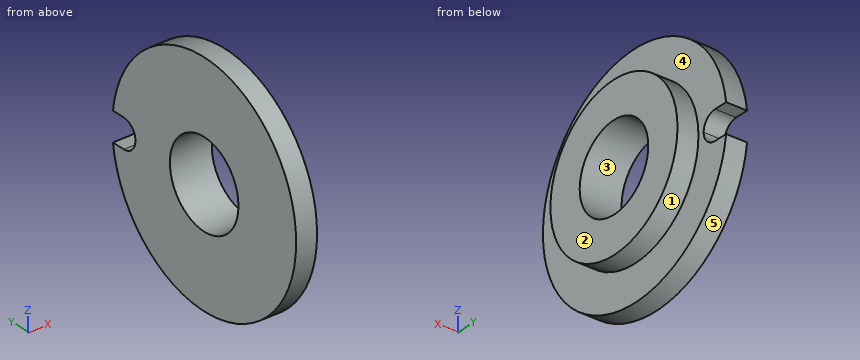
```python
from build123d import *

# Parameters (mm, degrees)
F0_R     = 11
F0_R_2   = 7.6
F1_DEPTH = 2
F2_DEPTH = 2
F3_R     = 4.1
F4_DEPTH = 25
F6_DEPTH = 5


# Not quite as in the source:
# - a feature names something its author has since deleted; it is built from what else it names


with BuildPart() as f1:
    # F0 (on Right) → F1 (new body)
    with BuildSketch(Plane.YZ):
        Circle(F0_R)
        Circle(F0_R_2, mode=Mode.SUBTRACT)
        Circle(F0_R_2)
    extrude(amount=-F1_DEPTH)

    # F0 (on Right) → F2 (join)
    with BuildSketch(Plane.YZ):
        Circle(F0_R_2)
    extrude(amount=F2_DEPTH)

    # F3 (on face) → F4 (cut)
    with BuildSketch(Plane(origin=(-2, 0, 0), x_dir=(0, -1, 0), z_dir=(-1, 0, 0))):
        Circle(F3_R)
    extrude(amount=-F4_DEPTH, mode=Mode.SUBTRACT)

    # F5 (on face) → F6 (cut)
    with BuildSketch(Plane(origin=(-2, 0, 0), x_dir=(0, -1, 0), z_dir=(-1, 0, 0))):
        with BuildLine():
            ThreePointArc((-10.9129812948, -1.3808835065), (-10.9999996004, -0.0029651094), (-10.9137241581, 1.375))
            Line((-10.9137241581, 1.375), (-11.6283151001, 1.375))
            Line((-11.6283151001, 1.375), (-11.6283151001, -1.3808835065))
            Line((-11.6283151001, -1.3808835065), (-10.9129812948, -1.3808835065))
        make_face()
        with BuildLine():
            Line((-9.6, -1.375), (-9.6, 1.375))
            ThreePointArc((-9.6, 1.375), (-10.975, 0), (-9.6, -1.375))
        make_face()
        with BuildLine():
            ThreePointArc((-9.6, -1.375), (-10.975, 0), (-9.6, 1.375))
            Line((-9.6, 1.375), (-10.9137241581, 1.375))
            ThreePointArc((-10.9137241581, 1.375), (-10.9999996004, -0.0029651094), (-10.9129812948, -1.3808835065))
            Line((-10.9129812948, -1.3808835065), (-9.6, -1.3808835065))
            Line((-9.6, -1.3808835065), (-9.6, -1.375))
        make_face()
        with BuildLine():
            ThreePointArc((-9.6, -1.375), (-8.6277281759, -0.9722718241), (-8.225, 0))
            ThreePointArc((-8.225, 0), (-8.6277281759, 0.9722718241), (-9.6, 1.375))
            Line((-9.6, 1.375), (-9.6, -1.375))
        make_face()
    extrude(amount=-F6_DEPTH, mode=Mode.SUBTRACT)


solid = f1.part
```
CAD build for the part. Positions are in the model's coordinates, mm. Face numbers are marked on the shaded views. A direction names the side the tool comes from. Round coordinates to 2 decimals unless told otherwise and drop trailing zeros. Write each loop counter-clockwise with the first axis right and the second up, starting at its lowest first coordinate (ties: lowest second). Pieces come first, ordered by that corner, then holes. Notation, with made-up numbers: (56.5, 63) -> (62.5, 63) arc R24 ccw to (62.5, 74) -> close; hole circle Ø7 at (78.25, -32.5). An arc over 180 degrees is marked (long way). Answer in a Markdown table with one row per item. Add a question column.
Item 1: Saw through at A-A, the plane y = 0. Write the cut outline in (x, z), then the cut area to 3 significant figures.
Item 2: Saw through at C-C, the plane y = 6.75. Write the cut outline in (x, z), then the cut area to 3 significant figures.
Item 3: Saw through at B-B, the plane x = -0.8. Write the cut outline in (y, z) (3 decimals), then the cut area to 3 significant figures.
Item 4: Saw through at D-D, the plane z = 6.5. Write the cut outline in (x, y).
Item 5: Drop flat-ended pins along their axis: pin 1 Ø4 at (y, z) = (6.5, -4) entering from +X; pin 2 Ø1.4 at (x, y) = (-1, 10) entering from -Z; pin 3 Ø1 at (x, z) = (-0.5, 8.5) entering from +Y. Give the stop position or say it passes through.
Item 6: Which spindle directions (+Z, -Z, +X, -X, +Y, -Y) get a long thin tool onto all of the face, cutting with end or side? Do the marked faces 1 and 2. Say none if no direction does.
Item 7: Mould opens along Y. For the marked faces 3, 4 and 5 say: pulls with the +Y half, pulls with the -Y half, needs draft (parallel to the pull), parting line crosses it, or undercut.
Item 8: Drill centre lines: line 1 (Z direction, x = -0.65, y = 0); line 2 (Z direction, x = 0.35, y = 0); line 3 (X direction, y = 0.5, z = 9). Where is each one in solid material? Low to high. Write a range as from..to.
Findings below:
| question | item | result |
|---|---|---|
| 1 | outline | (-2, -11) -> (0, -11) -> (0, -7.6) -> (2, -7.6) -> (2, -4.1) -> (-2, -4.1) -> close; (-2, 4.1) -> (2, 4.1) -> (2, 7.6) -> (0, 7.6) -> (0, 11) -> (-2, 11) -> close |
| 1 | area | 41.6 mm^2 |
| 2 | outline | (-2, -8.69) -> (0, -8.69) -> (0, -3.49) -> (2, -3.49) -> (2, 3.49) -> (0, 3.49) -> (0, 8.69) -> (-2, 8.69) -> close |
| 2 | area | 48.7 mm^2 |
| 3 | outline | (9.6, -1.381) -> (9.6, -1.375) arc R1.375 cw to (9.6, 1.375) -> (10.914, 1.375) arc R11 ccw (long way) to (10.913, -1.381) -> close; hole circle Ø8.2 at (0, 0) |
| 3 | area | 321 mm^2 |
| 4 | outline | (-2, -8.87) -> (0, -8.87) -> (0, -3.94) -> (2, -3.94) -> (2, 3.94) -> (0, 3.94) -> (0, 8.87) -> (-2, 8.87) -> close |
| 5 | pin 1 | stops at x = 2 |
| 5 | pin 2 | stops at z = -5.87 |
| 5 | pin 3 | stops at y = 7.55 |
| 6 | face 1 | +X |
| 6 | face 2 | +Z, -Z, +X, +Y, -Y |
| 7 | face 3 | undercut |
| 7 | face 4 | needs draft |
| 7 | face 5 | parting line crosses it |
| 8 | line 1 | z = -11..-4.1, 4.1..11 |
| 8 | line 2 | z = -7.6..-4.1, 4.1..7.6 |
| 8 | line 3 | x = -2..0 |
